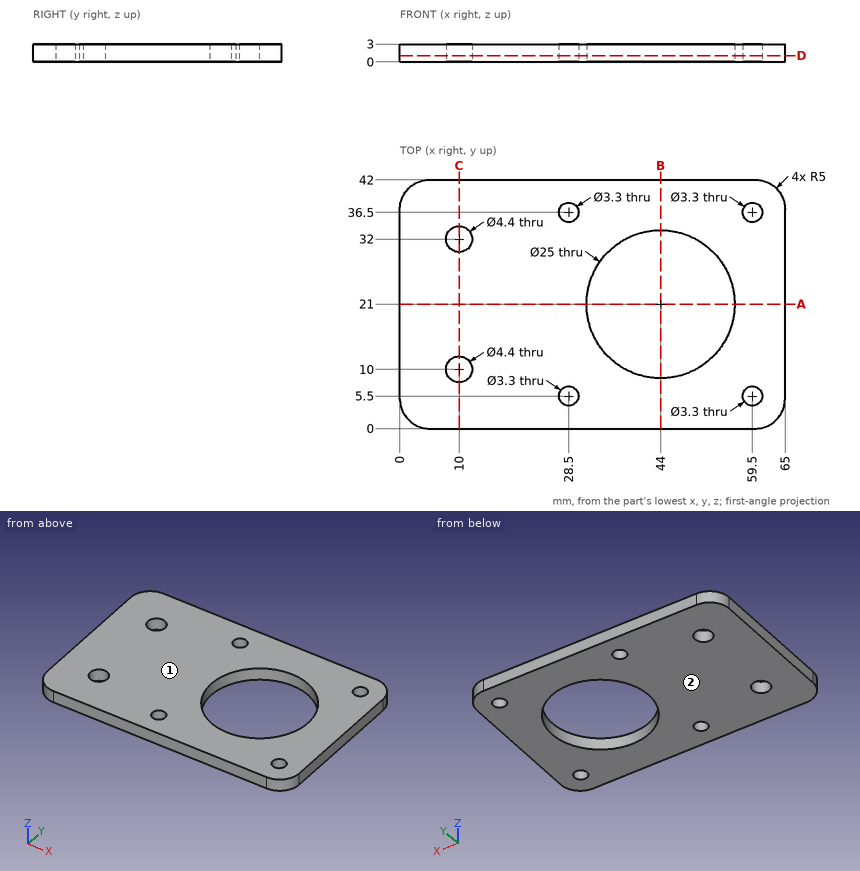
Part print with two shaded views. Sizes in mm from the minimum x, y, z corner. Give positions to 0.01 mm unless a question says otherwise; leave off trailing zeros. Loops run counter-clockwise (first coordinate to the right, second up) from the corner with the lowest first, then second, coordinate; pieces in that order, holes last. Notation, with made-up numbers: (-30, 47) - (-22, 47) arc R25 ccw to (-22, 80) - close; hole circle Ø5 at (11, -17). An arc over 180 degrees is marked (long way). Put each result on its own line as item: value.
Q1. Slice it at C-C (x = 10). Give the cut face in (y, z), plus the area to 3 significant figures.
Filled in:
outline: (0, 0) - (7.8, 0) - (7.8, 3) - (0, 3) - close; (12.2, 0) - (29.8, 0) - (29.8, 3) - (12.2, 3) - close; (34.2, 0) - (42, 0) - (42, 3) - (34.2, 3) - close
area: 99.6 mm²
Q2. Mould opens along Z. For the marked faces 1 and 2 say: pulls with the +Z half, pulls with the -Z half, needs draft (parallel to the pull), parting line crosses it, or undercut.
Filled in:
face 1: pulls with the +Z half
face 2: pulls with the -Z half
Q3. Slice it at B-B (x = 44). Give the cut face in (y, z), plus the area to 3 significant figures.
Filled in:
outline: (0, 0) - (8.5, 0) - (8.5, 3) - (0, 3) - close; (33.5, 0) - (42, 0) - (42, 3) - (33.5, 3) - close
area: 51.0 mm²
Q4. Probe line 1 along Y through (x, z) = (59.5, 1.5); line 2 along Y through (x, z) = (8.5, 1.95); line 3 along X through (y, z) = (21.5, 0.15). List the from-to ranges inside material, lowest first.
Filled in:
line 1: y = 0 to 3.85, 7.15 to 34.85, 38.15 to 42
line 2: y = 0 to 8.39, 11.61 to 30.39, 33.61 to 42
line 3: x = 0 to 31.51, 56.49 to 65
Q5. Slice it at A-A (y = 21). Give the cut face in (x, z).
Filled in:
outline: (0, 0) - (31.5, 0) - (31.5, 3) - (0, 3) - close; (56.5, 0) - (65, 0) - (65, 3) - (56.5, 3) - close
Q6. Slice it at D-D (z = 1.05). Give the cut face in (x, y), plus the area to 3 significant figures.
Filled in:
outline: (0, 5) arc R5 ccw to (5, 0) - (60, 0) arc R5 ccw to (65, 5) - (65, 37) arc R5 ccw to (60, 42) - (5, 42) arc R5 ccw to (0, 37) - close; hole circle Ø4.4 at (10, 10); hole circle Ø4.4 at (10, 32); hole circle Ø3.3 at (28.5, 5.5); hole circle Ø3.3 at (28.5, 36.5); hole circle Ø25 at (44, 21); hole circle Ø3.3 at (59.5, 5.5); hole circle Ø3.3 at (59.5, 36.5)
area: 2,150 mm²
